```python
from build123d import *

# Parameters (mm, degrees)
F0_R     = 2
F0_R_2   = 3.5
F0_R_3   = 2.25
F0_R_4   = 8.5
F0_R_5   = 13
F1_DEPTH = 8
F2_R     = 10


with BuildPart() as f1:
    # F0 (on Top) → F1 (new body)
    with BuildSketch(Plane.XY):
        with BuildLine():
            Line((0, 30), (0, 0))
            Line((0, 0), (120, 0))
            Line((120, 0), (120, 51.421356))
            Line((120, 51.421356), (-30, 201.421356))
            Line((-30, 201.421356), (-30, 300))
            Line((-30, 300), (-130, 300))
            Line((-130, 300), (-130, 290.75))
            Line((-130, 290.75), (-126, 290.75))
            ThreePointArc((-126, 290.75), (-122.75, 287.5), (-126, 284.25))
            Line((-126, 284.25), (-130, 284.25))
            Line((-130, 284.25), (-130, 275))
            Line((-130, 275), (-122, 275))
            Line((-122, 275), (-122, 250))
            Line((-122, 250), (-130, 250))
            Line((-130, 250), (-130, 240.75))
            Line((-130, 240.75), (-126, 240.75))
            ThreePointArc((-126, 240.75), (-122.75, 237.5), (-126, 234.25))
            Line((-126, 234.25), (-130, 234.25))
            Line((-130, 234.25), (-130, 160))
            Line((-130, 160), (0, 30))
        make_face()
        with Locations((7, 7)):
            Circle(F0_R, mode=Mode.SUBTRACT)
        with Locations((41, 7)):
            Circle(F0_R, mode=Mode.SUBTRACT)
        with Locations((7, 43)):
            Circle(F0_R, mode=Mode.SUBTRACT)
        with Locations((41, 43)):
            Circle(F0_R, mode=Mode.SUBTRACT)
        with Locations((60, 8)):
            Circle(F0_R_2, mode=Mode.SUBTRACT)
        with Locations((79, 7)):
            Circle(F0_R, mode=Mode.SUBTRACT)
        with Locations((113, 7)):
            Circle(F0_R, mode=Mode.SUBTRACT)
        with Locations((60, 40)):
            Circle(F0_R_2, mode=Mode.SUBTRACT)
        with Locations((79, 43)):
            Circle(F0_R, mode=Mode.SUBTRACT)
        with Locations((113, 43)):
            Circle(F0_R, mode=Mode.SUBTRACT)
        with Locations((-115, 190)):
            Circle(F0_R, mode=Mode.SUBTRACT)
        with Locations((-111.263456, 213.736544)):
            Circle(F0_R_3, mode=Mode.SUBTRACT)
        with Locations((-95, 190)):
            Circle(F0_R_4, mode=Mode.SUBTRACT)
        with Locations((-75, 190)):
            Circle(F0_R, mode=Mode.SUBTRACT)
        with Locations((-78.736544, 213.736544)):
            Circle(F0_R_3, mode=Mode.SUBTRACT)
        with Locations((-111.263456, 246.263456)):
            Circle(F0_R_3, mode=Mode.SUBTRACT)
        with Locations((-95, 230)):
            Circle(F0_R_5, mode=Mode.SUBTRACT)
        with Locations((-78.736544, 246.263456)):
            Circle(F0_R_3, mode=Mode.SUBTRACT)
        with Locations((-115, 270)):
            Circle(F0_R, mode=Mode.SUBTRACT)
        with Locations((-95, 270)):
            Circle(F0_R_4, mode=Mode.SUBTRACT)
        with Locations((-75, 270)):
            Circle(F0_R, mode=Mode.SUBTRACT)
    extrude(amount=F1_DEPTH)

    # F2
    f2_edges = [f1.edges().sort_by_distance(p)[0] for p in [
        (-30, 300, 4),
        (-30, 201.421356, 4),
        (-130, 160, 4),
        (0, 30, 4),
        (120, 51.421356, 4),
    ]]
    fillet(f2_edges, radius=F2_R)


solid = f1.part
```
Read the model definition and answer for the solid it produces. Units are mm, in the model's axes. A direction names the side the tool comes from. Round coordinates to 2 decimals unless told otherwise and drop trailing zeros. Write each loop counter-clockwise with the first axis right and the second up, starting at its lowest first coordinate (ties: lowest second). Pieces come first, ordered by that corner, then holes. Notation, with made-up numbers: (7.25, 24) - (15.25, 24) arc R10 cw to (15.25, 36) - close; hole circle Ø4 at (34, 59.25). An arc over 180 degrees is marked (long way). One line per item, written item: value.
Q1. Find section A-A (y = 230). Determine the outline of the cut face in (x, z).
The answers:
outline: (-130, 0) - (-108, 0) - (-108, 8) - (-130, 8) - close; (-82, 0) - (-30, 0) - (-30, 8) - (-82, 8) - close
Q2. Find section C-C (z = 5.75). Count the separate pieces of the cut face and the enclosed holes in it, and give its area (3 significant figures).
The answers:
separate pieces: 1
enclosed holes: 21
area: 35,000 mm2
Q3. Which of the six approach directions +Z, -Z, +X, -X, +Y, -Y give full straight-line access (tool end or side, diameter ignored) to faces 4 (the flat face through (0, 13, 4)), 5 (the flat face through (-35, 152, 8)), 6 (the flat face through (-126, 250, 4))?
The answers:
face 4: +Z, -Z, -X, -Y
face 5: +Z, +X, -X, +Y, -Y
face 6: +Z, -Z, -X
Q4. Each of these flat-tipped pins is pushed along its axis until it touches: P1, Ø1, axis at y = 253, z = 5, coming from the -X side; P2, Ø1, axis at x = -30.5, z = 3.5, coming from the -Y side; P3, Ø4, axis at y = 142, z = 7, coming from the -X side; P4, Ø7, axis at x = -78.74, y = 213.74, coming from the -Z side. Where does it stop, or does it pass through?
The answers:
P1: stops at x = -122
P2: stops at y = 60
P3: stops at x = -114
P4: stops at z = 0
Q5. For a pull along Y with two mould halves and no side action, classify faces 1 (the flat face through (46.01, 125.41, 3.94)), 2 (the flat face through (-122, 263, 4)), 3 (the flat face through (-130, 200, 4)) as pulls with the +Y half, pulls with the -Y half, needs draft (parallel to the pull), parting line crosses it, or undercut.
The answers:
face 1: pulls with the +Y half
face 2: undercut
face 3: needs draft
Q6. Straight lines are drawn through the part: line 1 (Y direction, x = -90, z = 4); line 2 (Y direction, x = 7, z = 2.5); line 3 (X direction, y = 17, z = 7.75). For each, find the intervals that lie inside material, in ascending order. Write a range as from..to.
The answers:
line 1: y = 120..183.13, 196.87..218, 242..263.13, 276.87..300
line 2: y = 0..5, 9..41, 45..164.42
line 3: x = 0..120
Q7. Find section B-B (x = 60). Determine the outline of the cut face in (y, z).
The answers:
outline: (0, 0) - (4.5, 0) - (4.5, 8) - (0, 8) - close; (11.5, 0) - (36.5, 0) - (36.5, 8) - (11.5, 8) - close; (43.5, 0) - (111.42, 0) - (111.42, 8) - (43.5, 8) - close
Q8. Find section D-D (y = 67.5). Determine the outline of the cut face in (x, z), and give its area (3 significant figures).
The answers:
outline: (-37.5, 0) - (103.92, 0) - (103.92, 8) - (-37.5, 8) - close
area: 1,130 mm2
